Autodesk Inventor part; units mm, degrees
ref_plane "Work Plane1" through (0, 431, 0) normal (0, 1, 0) x (-1, 0, 0)
ref_plane "YZ Plane" through (0, 0, 0) normal (1, 0, 0) x (0, 1, 0)
ref_plane "XY Plane" through (0, 0, 0) normal (0, 0, 1) x (1, 0, 0)
ref_plane "Work Plane1" through (0, 431, 0) normal (0, 1, 0) x (-1, 0, 0)
sketch "Sketch1" plane through (0, 431, 0) normal (0, 1, 0) x (-1, 0, 0)
  line L0 (-54.5291, -19.1661) -> (-51.4685, -22.2268)
  line L1 (-67.4685, 2.2039) -> (-67.4685, -12.5361)
  line L2 (-51.4685, 11.8946) -> (-54.5291, 8.8339)
  line L3 (-48.9685, -9.1661) -> (-48.9685, -12.5361)
  line L4 (-64.5291, -1.1661) -> (-65.9685, -1.1661)
  line L5 (-54.8385, 14.8339) -> (-54.8385, 13.3339)
  line L6 (-63.4685, -23.6661) -> (-63.4685, -22.2268)
  line L7 (-53.4685, -18.1054) -> (-53.4685, -12.2268)
  line L8 (-67.4685, -25.1661) -> (-60.0985, -25.1661)
  line L9 (-48.9685, 7.4639) -> (-47.4685, 7.4639)
  line L10 (-63.4685, -2.2268) -> (-60.4078, 0.8339)
  line L11 (-48.9685, -17.7961) -> (-48.9685, -21.1661)
  line L12 (-64.5291, 10.8339) -> (-61.4685, 7.7732)
  line L13 (-53.4685, 7.7732) -> (-50.4078, 10.8339)
  line L14 (-54.5291, -11.1661) -> (-60.4078, -11.1661)
  line L15 (-65.9685, -21.1661) -> (-65.9685, -17.7961)
  line L16 (-67.4685, 7.4639) -> (-65.9685, 7.4639)
  line L17 (-60.0985, 13.3339) -> (-60.0985, 14.8339)
  line L18 (-61.4685, -12.2268) -> (-61.4685, -18.1054)
  line L19 (-47.4685, -25.1661) -> (-47.4685, -17.7961)
  line L20 (-48.9685, -1.1661) -> (-50.4078, -1.1661)
  line L21 (-47.4685, -12.5361) -> (-47.4685, 2.2039)
  line L22 (-51.4685, -23.6661) -> (-54.8385, -23.6661)
  line L23 (-65.9685, -12.5361) -> (-65.9685, -9.1661)
  line L24 (-60.4078, 8.8339) -> (-63.4685, 11.8946)
  line L25 (-50.4078, -9.1661) -> (-48.9685, -9.1661)
  line L26 (-51.4685, 13.3339) -> (-51.4685, 11.8946)
  line L27 (-60.4078, -19.1661) -> (-54.5291, -19.1661)
  line L28 (-65.9685, 2.2039) -> (-67.4685, 2.2039)
  line L29 (-50.4078, -21.1661) -> (-53.4685, -18.1054)
  line L30 (-47.4685, 14.8339) -> (-54.8385, 14.8339)
  line L31 (-61.4685, 1.8946) -> (-64.5291, -1.1661)
  line L32 (-54.5291, 0.8339) -> (-51.4685, -2.2268)
  line L33 (-60.0985, -23.6661) -> (-63.4685, -23.6661)
  line L34 (-67.4685, -17.7961) -> (-67.4685, -25.1661)
  line L35 (-65.9685, 10.8339) -> (-64.5291, 10.8339)
  line L36 (-47.4685, -17.7961) -> (-48.9685, -17.7961)
  line L37 (-48.9685, 10.8339) -> (-48.9685, 7.4639)
  line L38 (-63.4685, -8.1054) -> (-63.4685, -2.2268)
  line L39 (-53.4685, 1.8946) -> (-53.4685, 7.7732)
  line L40 (-51.4685, -8.1054) -> (-54.5291, -11.1661)
  line L41 (-67.4685, 14.8339) -> (-67.4685, 7.4639)
  line L42 (-64.5291, -21.1661) -> (-65.9685, -21.1661)
  line L43 (-54.8385, -25.1661) -> (-47.4685, -25.1661)
  line L44 (-63.4685, 13.3339) -> (-60.0985, 13.3339)
  line L45 (-48.9685, 2.2039) -> (-48.9685, -1.1661)
  line L46 (-64.5291, -9.1661) -> (-61.4685, -12.2268)
  line L47 (-51.4685, -22.2268) -> (-51.4685, -23.6661)
  line L48 (-48.9685, -12.5361) -> (-47.4685, -12.5361)
  line L49 (-67.4685, -12.5361) -> (-65.9685, -12.5361)
  line L50 (-54.5291, 8.8339) -> (-60.4078, 8.8339)
  line L51 (-65.9685, -1.1661) -> (-65.9685, 2.2039)
  line L52 (-53.4685, -12.2268) -> (-50.4078, -9.1661)
  line L53 (-54.8385, 13.3339) -> (-51.4685, 13.3339)
  line L54 (-63.4685, -22.2268) -> (-60.4078, -19.1661)
  line L55 (-47.4685, 7.4639) -> (-47.4685, 14.8339)
  line L56 (-60.4078, 0.8339) -> (-54.5291, 0.8339)
  line L57 (-48.9685, -21.1661) -> (-50.4078, -21.1661)
  line L58 (-61.4685, 7.7732) -> (-61.4685, 1.8946)
  line L59 (-60.0985, -25.1661) -> (-60.0985, -23.6661)
  line L60 (-60.4078, -11.1661) -> (-63.4685, -8.1054)
  line L61 (-65.9685, 7.4639) -> (-65.9685, 10.8339)
  line L62 (-50.4078, 10.8339) -> (-48.9685, 10.8339)
  line L63 (-65.9685, -17.7961) -> (-67.4685, -17.7961)
  line L64 (-50.4078, -1.1661) -> (-53.4685, 1.8946)
  line L65 (-61.4685, -18.1054) -> (-64.5291, -21.1661)
  line L66 (-51.4685, -2.2268) -> (-51.4685, -8.1054)
  line L67 (-60.0985, 14.8339) -> (-67.4685, 14.8339)
  line L68 (-54.8385, -23.6661) -> (-54.8385, -25.1661)
  line L69 (-63.4685, 11.8946) -> (-63.4685, 13.3339)
  line L70 (-65.9685, -9.1661) -> (-64.5291, -9.1661)
  line L71 (-47.4685, 2.2039) -> (-48.9685, 2.2039)
extrude "Extrusion1" add sketch "Sketch1" against normal blind 431
hole "Hole2" at (57.4685, 431, 4.8339) direction (0, -1, 0) diameter 4 depth 431
sketch "Sketch2" plane through (0, 431, 0) normal (0, 1, 0) x (-1, 0, 0)
  point P0 (-57.4685, 4.8339)
hole "Hole1" at (57.4685, 431, -15.1661) direction (0, -1, 0) diameter 4 depth 431
sketch "Sketch3" plane through (0, 431, 0) normal (0, 1, 0) x (-1, 0, 0)
  point P0 (-57.4685, -15.1661)
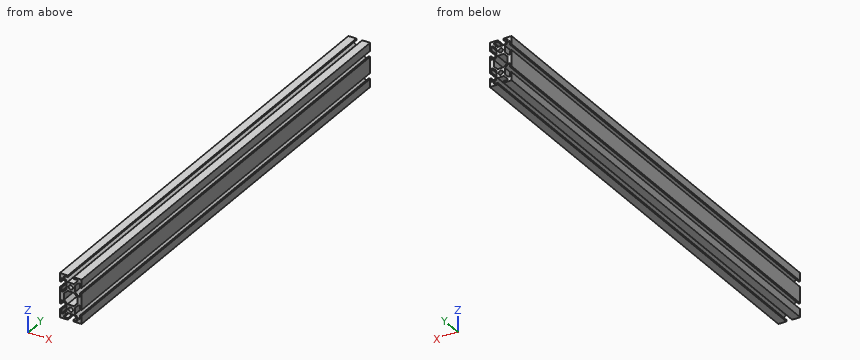
Check sheet for the modelled part. Datum: model origin and axes. Units: mm. Round coordinates to 2 decimals unless told otherwise and drop trailing zeros. Answer as a JSON object with one key per item and string values. Group by question number.
Q1. Sectioned sample at A-A, the plane y = 304. Count the separate pieces of the cut face and the enclosed holes in it, plus the area to 3 significant figures.
Q2. Scan lines: line 1 along Z through (x, y) = (57.5, 133.5); line 2 along Z through (x, y) = (48.5, 377); line 3 along Z through (x, y) = (54.5, 150). Record each from-to range of solid material in increasing order. Write a range as [from, to].
Q3. Gauge pin test, flat end, axial feed: P1, Ø1.8, axis at x = 58, y = 241, coming from the -Z side. Record the tip position at first contact, or that the pin passes through.
Solution:
{
 "1": {"separate pieces": "1", "enclosed holes": "3", "area": "334 mm²"},
 "2": {"line 1": "z = [-19.17, -17.17], [-13.17, -11.17], [0.83, 2.83], [6.83, 8.83]", "line 2": "z = [-25.17, -17.8], [-12.54, 2.2], [7.46, 14.83]", "line 3": "z = [-25.17, -23.67], [-19.2, -11.14], [0.8, 8.86], [13.33, 14.83]"},
 "3": {"P1": "stops at z = -19.17"}
}
